Check sheet for the drawn part. Datum: minimum x, y, z corner. Units: mm. A direction names the side the tool comes from. Coordinates: 2 decimals unless noted, no trailing zeros. Write each loop counter-clockwise with the first axis right and the second up, starting at its lowest first coordinate (ties: lowest second). Pieces come first, ordered by that corner, then holes. Notation, with made-up numbers: M -0.5,32 L 16.5,32 A12 cw 16.5,39 Z; hole C -14.75,66 d1. An arc over 180 degrees is marked long. Answer as a JSON object with one key per item and string values. Group by question number.
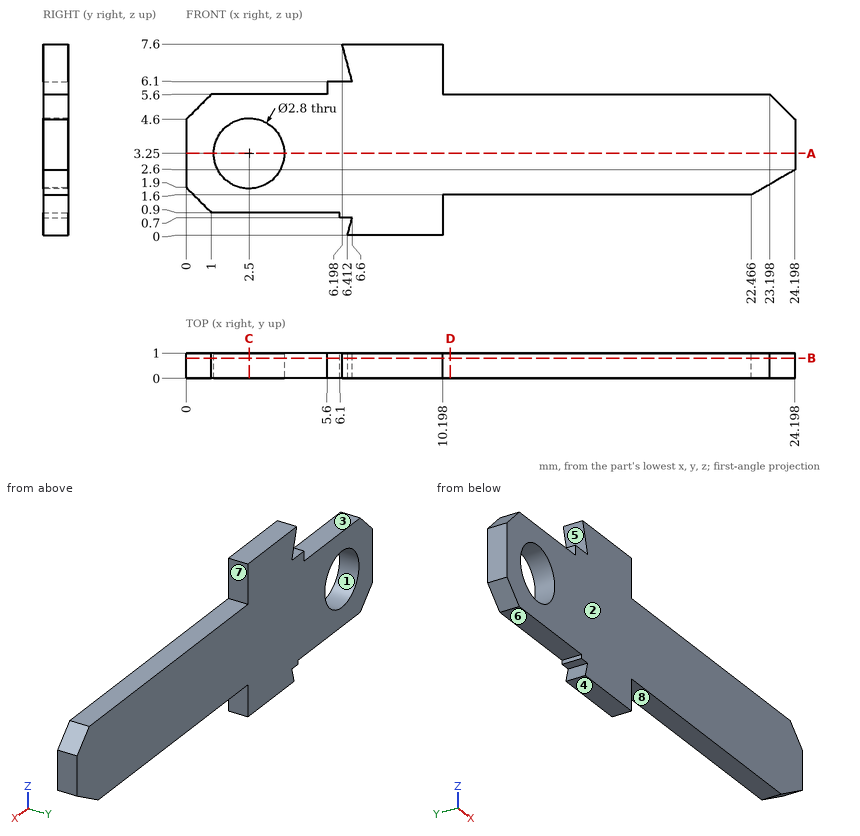
1) Set-up check for the marked faces 4, 5, 6, 7 and 8: record each of +Z, -Z, +X, -X, +Y, -Y from which the full face is reachable in a straight line by a thin tool's end or side.
2) Go/stop test with flat-tipped pins: pin 1 Ø0.5 at (y, z) = (0.5, 6.5) entering from +X; pin 2 Ø0.5 at (x, y) = (17.5, 0.5) entering from -Z; pin 3 Ø0.6 at (y, z) = (0.5, 6) entering from -X. Record where each tip stops, or that it passes through.
3) Section check C-C (x = 2.5). Record the cut outline in (y, z).
4) Section check B-B (y = 0.8). Record the cut outline in (x, z).
5) Draft check along Z on the marked faces 1, 2 and 3. Enter one of: +Z half, -Z half, draft (parallel to the pull), parting line (faces both ways), or undercut.
6) Section check D-D (x = 10.5). Record the cut outline in (y, z).
7) Material ranges on probe 1 along Z at (x, y) = (2.5, 0.3); probe 2 along Z at (x, y) = (18, 0.85); probe 3 along X at (y, z) = (0.9, 3.5), recorded low to high. Write a range as [from, to].
8) Section check A-A (z = 3.25). Record the cut outline in (x, y), then the cut area to 3 significant figures.
Entries:
{
 "1": {"face 4": "-Z, +X, -X, +Y, -Y", "face 5": "-X, +Y, -Y", "face 6": "-Z, -X, +Y, -Y", "face 7": "+Z, +X, +Y, -Y", "face 8": "-Z, +X, +Y, -Y"},
 "2": {"pin 1": "x = 10.2", "pin 2": "z = 1.6", "pin 3": "x = 5.6"},
 "3": {"outline": "M 0,0.9 L 1,0.9 L 1,1.85 L 0,1.85 Z; M 0,4.65 L 1,4.65 L 1,5.6 L 0,5.6 Z"},
 "4": {"outline": "M 0,1.9 L 1,0.9 L 6.1,0.9 L 6.1,0.7 L 6.6,0.7 L 6.41,0 L 10.2,0 L 10.2,1.6 L 22.47,1.6 L 24.2,2.6 L 24.2,4.6 L 23.2,5.6 L 10.2,5.6 L 10.2,7.6 L 6.2,7.6 L 6.6,6.1 L 5.6,6.1 L 5.6,5.6 L 1,5.6 L 0,4.6 Z; hole C 2.5,3.25 d2.8"},
 "5": {"face 1": "undercut", "face 2": "draft", "face 3": "+Z half"},
 "6": {"outline": "M 0,1.6 L 1,1.6 L 1,5.6 L 0,5.6 Z"},
 "7": {"probe 1": "[0.9, 1.85], [4.65, 5.6]", "probe 2": "[1.6, 5.6]", "probe 3": "[0, 1.12], [3.88, 24.2]"},
 "8": {"outline": "M 0,0 L 1.1,0 L 1.1,1 L 0,1 Z; M 3.9,0 L 24.2,0 L 24.2,1 L 3.9,1 Z", "area": "21.4 mm^2"}
}
